The listing builds one solid part. Answer for the finished solid, in the listing's coordinates (mm). Coordinates: 2 decimals unless noted, no trailing zeros. Order: outer loops, then holes, each group sorted by start corner. A loop starts at its lowest first (then second) coordinate and runs counter-clockwise, first axis right, second up.
from build123d import *

# Parameters (mm, degrees)
ESQUISSE1_R          = 5
ESQUISSE1_R_2        = 2
BASE_EXTRUSION_DEPTH = 20
CHANFREIN1_SIZE      = 1
CHANFREIN2_SIZE      = 0.5


with BuildPart() as part:
    # Esquisse1 → Base-Extrusion (new body)
    with BuildSketch(Plane.XY):
        Circle(ESQUISSE1_R)
        Circle(ESQUISSE1_R_2, mode=Mode.SUBTRACT)
    extrude(amount=BASE_EXTRUSION_DEPTH)

    # Chanfrein1
    chanfrein1_edges = [part.edges().sort_by_distance(p)[0] for p in [
        (-5, 0, 0),
        (-5, 0, 20),
    ]]
    chamfer(chanfrein1_edges, length=CHANFREIN1_SIZE)

    # Chanfrein2
    chanfrein2_edges = [part.edges().sort_by_distance(p)[0] for p in [
        (-2, 0, 0),
        (-2, 0, 20),
    ]]
    chamfer(chanfrein2_edges, length=CHANFREIN2_SIZE)


solid = part.part
(1) Find section A-A on y = 0. Determine the outline of the cut face in (x, z), then the cut area to 4 significant figures.
(2) Find the intervals of material crossed by probe 1 along Y at (x, z) = (0, 6); probe 2 along Y at (x, z) = (-1.25, 8); probe 3 along X at (y, z) = (1.5, 5.25), in increasing order.
(3) Find section C-C on z = 6.25. Determine the outline of the cut face in (x, y), then the cut area to 3 significant figures.
(4) Given pin 1 Ø1.5 at (y, z) = (-3.5, 2.5) entering from -X; pin 2 Ø5 at (x, z) = (3.5, 12) entering from -Y, each flat-ended and moving along its own axis, determine where each tip first touches the part or whether it passes through.
(5) The mould has two halves that part along Y. Classify faces 1 (the cylindrical face through (0, -2, 10)), 2 (the flat face through (2, 2, 20)), 3 (the cylindrical face through (-1.08, -4.88, 9.87)): pulls with the +Y half, pulls with the -Y half, needs draft (parallel to the pull), parting line crosses it, or undercut.
Resolved:
1. outline: (-5, 1) - (-4, 0) - (-2.5, 0) - (-2, 0.5) - (-2, 19.5) - (-2.5, 20) - (-4, 20) - (-5, 19) - close; (2, 0.5) - (2.5, 0) - (4, 0) - (5, 1) - (5, 19) - (4, 20) - (2.5, 20) - (2, 19.5) - close
1. area: 117.5 mm2
2. probe 1: y = -5 to -2, 2 to 5
2. probe 2: y = -4.84 to -1.56, 1.56 to 4.84
2. probe 3: x = -4.77 to -1.32, 1.32 to 4.77
3. outline: circle Ø10 at (0, 0); hole circle Ø4 at (0, 0)
3. area: 66.0 mm2
4. pin 1: stops at x = -4.18
4. pin 2: stops at y = -4.9
5. face 1: undercut
5. face 2: needs draft
5. face 3: parting line crosses it
